```python
from build123d import *

# Parameters (mm, degrees)
SKETCH1_W                                       = 127.7
SKETCH1_H                                       = 87.4
BOSS_EXTRUDE1_DEPTH                             = 39.5
SHELL1_T                                        = -3
FILLET2_R                                       = 4
CSK_FOR_M2_FLAT_HEAD_MACHINE_SCREW3_D           = 3
CSK_FOR_M2_FLAT_HEAD_MACHINE_SCREW3_CSINK_D     = 5.4
CSK_FOR_M2_FLAT_HEAD_MACHINE_SCREW3_CSINK_ANGLE = 90
CUT_EXTRUDE1_REACH                              = 89.4
CHAMFER1_SIZE                                   = 1
CHAMFER2_SIZE                                   = 1
CHAMFER3_SIZE                                   = 1


with BuildPart() as part:
    # Sketch1 → Boss-Extrude1 (new body)
    with BuildSketch(Plane(origin=(0, 0, 0), x_dir=(1, 0, 0), z_dir=(0, 1, 0))):
        Rectangle(SKETCH1_W, SKETCH1_H)
    extrude(amount=BOSS_EXTRUDE1_DEPTH)

    # Shell1
    shell1_openings = [part.faces().sort_by_distance(p)[0] for p in [
        (0, 0, 0),
    ]]
    offset(amount=SHELL1_T, openings=shell1_openings, kind=Kind.INTERSECTION)

    # Fillet2
    fillet2_edges = [part.edges().sort_by_distance(p)[0] for p in [
        (-63.85, 19.75, -43.7),
        (63.85, 19.75, -43.7),
        (63.85, 19.75, 43.7),
        (-63.85, 19.75, 43.7),
    ]]
    fillet(fillet2_edges, radius=FILLET2_R)

    # CSK for M2 Flat Head Machine Screw3 (through all)
    with Locations(Plane(origin=(56.4, 39.5, -33.4), x_dir=(0, 0, 1), z_dir=(0, 1, 0))):
        with Locations((0, 0), (0, -113), (65.8, -113), (65.8, 0)):
            CounterSinkHole(CSK_FOR_M2_FLAT_HEAD_MACHINE_SCREW3_D / 2, CSK_FOR_M2_FLAT_HEAD_MACHINE_SCREW3_CSINK_D / 2, counter_sink_angle=CSK_FOR_M2_FLAT_HEAD_MACHINE_SCREW3_CSINK_ANGLE)

    # Sketch9 → Cut-Extrude1 (cut, up to next)
    with BuildSketch(Plane(origin=(0, 0, -43.7), x_dir=(-1, 0, 0), z_dir=(0, 0, -1)), mode=Mode.PRIVATE) as cut_extrude1_sk1:
        with BuildLine():
            Line((-27.2, 22.11), (-22.5, 22.11))
            ThreePointArc((-22.5, 22.11), (-18.75, 18.36), (-22.5, 14.61))
            Line((-22.5, 14.61), (-27.2, 14.61))
            ThreePointArc((-27.2, 14.61), (-30.95, 18.36), (-27.2, 22.11))
        make_face()
    cut_extrude1_tool1 = extrude(cut_extrude1_sk1.sketch, amount=-CUT_EXTRUDE1_REACH, mode=Mode.PRIVATE) & part.part
    add(cut_extrude1_tool1.solids().sort_by_distance((24.85, 18.36, -43.7))[0], mode=Mode.SUBTRACT)

    # Chamfer1
    chamfer1_edges = [part.edges().sort_by_distance(p)[0] for p in [
        (30.95, 18.36, -43.7),
        (24.85, 14.61, -43.7),
        (18.75, 18.36, -43.7),
        (24.85, 22.11, -43.7),
        (24.85, 14.61, -40.7),
        (18.75, 18.36, -40.7),
        (24.85, 22.11, -40.7),
        (30.95, 18.36, -40.7),
    ]]
    chamfer(chamfer1_edges, length=CHAMFER1_SIZE)

    # Chamfer2
    chamfer2_edges = [part.edges().sort_by_distance(p)[0] for p in [
        (0, 39.5, -43.7),
        (63.85, 39.5, 0),
        (-63.85, 39.5, 0),
        (0, 39.5, 43.7),
        (62.678427125, 39.5, 42.528427125),
        (-62.678427125, 39.5, 42.528427125),
        (-62.678427125, 39.5, -42.528427125),
        (62.678427125, 39.5, -42.528427125),
    ]]
    chamfer(chamfer2_edges, length=CHAMFER2_SIZE)

    # Chamfer3
    chamfer3_edges = [part.edges().sort_by_distance(p)[0] for p in [
        (-60.85, 18.25, -40.7),
        (-60.85, 18.25, 40.7),
        (60.85, 18.25, 40.7),
        (60.85, 18.25, -40.7),
        (-60.85, 36.5, 0),
        (0, 36.5, 40.7),
        (60.85, 36.5, 0),
        (0, 36.5, -40.7),
    ]]
    chamfer(chamfer3_edges, length=CHAMFER3_SIZE)


solid = part.part
```
CAD build for the part. Positions are in the model's coordinates, mm. A direction names the side the tool comes from. Coordinates: 2 decimals unless noted, no trailing zeros. Order: outer loops, then holes, each group sorted by start corner. A loop starts at its lowest first (then second) coordinate and runs counter-clockwise, first axis right, second up. Notation, with made-up numbers: M -0.75,-20.75 L 36.25,-20.75 A18 cw 36.25,-12.75 Z; hole C -36,-34 d2. An arc over 180 degrees is marked long. Answer as CSV lines item,"result".
1) Cut at B-B (x = 56.4). List the corners of the cut face in (y, z), then the cut area to 3 significant figures.
Verdict:
outline,"M 0,-43.7 L 38.5,-43.7 L 39.5,-42.7 L 39.5,-36.1 L 38.3,-34.9 L 36.5,-34.9 L 36.5,-39.7 L 35.5,-40.7 L 0,-40.7 Z; M 0,40.7 L 35.5,40.7 L 36.5,39.7 L 36.5,33.9 L 38.3,33.9 L 39.5,35.1 L 39.5,42.7 L 38.5,43.7 L 0,43.7 Z; M 36.5,-31.9 L 38.3,-31.9 L 39.5,-30.7 L 39.5,29.7 L 38.3,30.9 L 36.5,30.9 Z"
area,"460 mm2"
2) 3-axis set-ups, long thin cutter, end or side, ignore diameter. For faces 4 (the conical face through (18.59, 18.27, -41.54)), 5 (the flat face through (-1, 18, -40.7)), 6 (the conical face through (31.11, 18.27, -42.86)): which of +Z, -Z, +X, -X, +Y, -Y reach the whole face in a straight line?
Verdict:
face 4,"none"
face 5,"-Y"
face 6,"-Z"
3) Flat gauge pins, fed straight in: P1, Ø5, axis at x = -56.6, z = 32.4, coming from the -Y side; P2, Ø2.5, axis at x = 56.4, z = 32.4, coming from the -Y side. Where does each tip first touch, or does it go through?
Verdict:
P1,"y = 36.5"
P2,"through"
4) Cut at D-D (x = 9.5). List the corners of the cut face in (y, z), then the cut area to 3 significant figures.
Verdict:
outline,"M 0,-43.7 L 38.5,-43.7 L 39.5,-42.7 L 39.5,42.7 L 38.5,43.7 L 0,43.7 L 0,40.7 L 35.5,40.7 L 36.5,39.7 L 36.5,-39.7 L 35.5,-40.7 L 0,-40.7 Z"
area,"481 mm2"
5) Cut at A-A (z = 32.4). List the corners of the cut face in (x, y), then the cut area to 3 significant figures.
Verdict:
outline,"M -63.85,0 L -60.85,0 L -60.85,35.5 L -59.85,36.5 L -58.1,36.5 L -58.1,38.3 L -59.3,39.5 L -62.85,39.5 L -63.85,38.5 Z; M -55.1,36.5 L 54.9,36.5 L 54.9,38.3 L 53.7,39.5 L -53.9,39.5 L -55.1,38.3 Z; M 57.9,36.5 L 59.85,36.5 L 60.85,35.5 L 60.85,0 L 63.85,0 L 63.85,38.5 L 62.85,39.5 L 59.1,39.5 L 57.9,38.3 Z"
area,"581 mm2"
6) Drill centre lines: L1, parallel to X at y = 37.4, z = -33.4; L2, parallel to Z at x = -56.6, y = 37.45; L3, parallel to X at y = 10, z = -38. Where is each one in solid material? Low to high. Write a range as from..to.
Verdict:
L1,"-63.85..-58.1, -55.1..54.9, 57.9..63.85"
L2,"-43.7..-34.9, -31.9..30.9, 33.9..43.7"
L3,"-63.85..-60.85, 60.85..63.85"
7) Mould opens along X. For faces 1 (the cylindrical face through (-62.709, 19.52, -42.497)), 2 (the cylindrical face through (-55.335, 37.387, -34.206)), 3 (the conical face through (62.137, 39.229, -42.038)) say: released by +X, released by -X, zero draft, split by the parting line, or undercut.
Verdict:
face 1,"released by -X"
face 2,"undercut"
face 3,"released by +X"
8) Cut at C-C (y = 29). List the corners of the cut face in (x, z), then the cut area to 3 significant figures.
Verdict:
outline,"M -63.85,-39.7 A4 ccw -59.85,-43.7 L 59.85,-43.7 A4 ccw 63.85,-39.7 L 63.85,39.7 A4 ccw 59.85,43.7 L -59.85,43.7 A4 ccw -63.85,39.7 Z; hole M -60.85,-39.7 L -59.85,-40.7 L 59.85,-40.7 L 60.85,-39.7 L 60.85,39.7 L 59.85,40.7 L -59.85,40.7 L -60.85,39.7 Z"
area,"1,240 mm2"
